Part model, mm, in its own coordinate system. Face numbers are marked on the shaded views. A direction names the side the tool comes from. Coordinates: 2 decimals unless noted, no trailing zeros. Write each loop counter-clockwise with the first axis right and the second up, starting at its lowest first coordinate (ties: lowest second). Pieces come first, ordered by that corner, then holes. Notation, with made-up numbers: (-21, -35.5) - (12, -35.5) arc R17 ccw to (12, -22.5) - close; hole circle Ø3 at (82.5, 65.25). An arc over 180 degrees is marked (long way). Use one line per item in the form item = value. Start each with the question number.
from build123d import *

# Parameters (mm, degrees)
BOSS_EXTRUDE1_OUTLINE_R = 28
BOSS_EXTRUDE1_DEPTH     = 3
BOSS_EXTRUDE3_START     = 20
BOSS_EXTRUDE3_DEPTH     = 20


# Read off the part's stored shape, not the designer's step: Boss-Extrude1
with BuildPart() as part:
    # Boss-Extrude1 outline → Boss-Extrude1 (new body)
    with BuildSketch(Plane.XY):
        with BuildLine():
            Line((30, -70), (30, 0))
            add(Edge.make_bspline(
                [(30, 0), (30, 122.919601085), (65, 122.919601085), (65, 152.5)],
                knots=[0, 0, 0, 0, 1, 1, 1, 1], degree=3))
            ThreePointArc((65, 152.5), (56.213203436, 173.713203436), (35, 182.5))
            add(Edge.make_bspline(
                [(-30, 0), (-30, 182.5), (35, 182.5)],
                knots=[0, 0, 0, 1, 1, 1], degree=2))
            Line((-30, 0), (-30, -70))
            Line((-30, -70), (30, -70))
        make_face()
        with Locations((0, -40)):
            Circle(BOSS_EXTRUDE1_OUTLINE_R, mode=Mode.SUBTRACT)
        with Locations((35, 152.5)):
            Circle(BOSS_EXTRUDE1_OUTLINE_R, mode=Mode.SUBTRACT)
    extrude(amount=BOSS_EXTRUDE1_DEPTH)

    # Sketch3 → Boss-Extrude3 (add)
    with BuildSketch(Plane(origin=(0, 0, 0), x_dir=(-1, 0, 0), z_dir=(0, 0, -1)).offset(BOSS_EXTRUDE3_START)):
        with BuildLine():
            Line((-30, 0), (-30, -70))
            Line((-30, -70), (30, -70))
            Line((30, -70), (30, 0))
            add(Edge.make_bspline(
                [(30, 0), (30, 182.5), (-35, 182.5)],
                knots=[0, 0, 0, 1, 1, 1], degree=2))
            ThreePointArc((-35, 182.5), (-56.213203436, 173.713203436), (-65, 152.5))
            add(Edge.make_bspline(
                [(-65, 152.5), (-65, 122.919601085), (-30, 122.919601085), (-30, 0)],
                knots=[0, 0, 0, 0, 1, 1, 1, 1], degree=3))
        make_face()
        with BuildLine():
            Line((-28, 0), (-28, -68))
            Line((-28, -68), (28, -68))
            Line((28, -68), (28, 0))
            add(Edge.make_bspline(
                [(28, 0), (28, 1.882428306), (27.9894412, 5.668914661), (27.926096555, 13.06867177), (27.76775639, 22.113138456), (27.45115367, 32.600472774), (26.860323994, 46.108658024), (25.805698034, 62.096829622), (24.035349894, 79.847577378), (21.76158749, 96.16063855), (18.061595292, 115.991158762), (12.190733374, 137.171036702), (3.196896645, 156.784444582), (-5.834661566, 168.281935437), (-13.924397363, 174.636152769), (-19.34693601, 177.454327423), (-23.921129202, 179.03154511), (-27.474819646, 179.877405657), (-30.546503211, 180.301515997), (-33.065469046, 180.471580895), (-34.357731157, 180.5), (-35, 180.5)],
                knots=[0.49382409, 0.49382409, 0.49382409, 0.49382409, 0.49393283, 0.494041569, 0.494259049, 0.494476528, 0.494694008, 0.495128967, 0.495563926, 0.495998885, 0.496433844, 0.497303761, 0.498173679, 0.499043597, 0.499478556, 0.499913515, 0.500130995, 0.500348474, 0.500565954, 0.500674693, 0.500783433, 0.500783433, 0.500783433, 0.500783433], degree=3))
            ThreePointArc((-35, 180.5), (-54.798989873, 172.298989873), (-63, 152.5))
            add(Edge.make_bspline(
                [(-63, 152.5), (-63, 152.069757812), (-62.983825045, 151.199286285), (-62.88918488, 149.540019878), (-62.658452593, 147.549741818), (-62.213886299, 145.2784002), (-61.410812146, 142.352354087), (-60.033210568, 138.80365362), (-57.846222702, 134.475175879), (-55.208976195, 129.863823008), (-51.231452034, 123.063969133), (-46.792456906, 114.875371889), (-42.352360132, 104.461715313), (-39.130632465, 95.326409045), (-36.123020534, 84.651250359), (-33.432349584, 72.218369024), (-31.538773259, 60.209244421), (-30.283559802, 49.501788472), (-29.484585221, 40.893227078), (-28.840668199, 31.678686061), (-28.443815603, 23.471810433), (-28.216507678, 16.574966065), (-28.092697498, 11.23438398), (-28.029735078, 6.636857178), (-28.004285655, 2.878237886), (-28, 0.955822894), (-28, 0)],
                knots=[0, 0, 0, 0, 0.015625, 0.03125, 0.0625, 0.09375, 0.125, 0.1875, 0.25, 0.3125, 0.375, 0.5, 0.5625, 0.625, 0.6875, 0.75, 0.8125, 0.84375, 0.875, 0.90625, 0.9375, 0.953125, 0.96875, 0.984375, 0.9921875, 1, 1, 1, 1], degree=3))
        make_face(mode=Mode.SUBTRACT)
    extrude(amount=-BOSS_EXTRUDE3_DEPTH)


solid = part.part
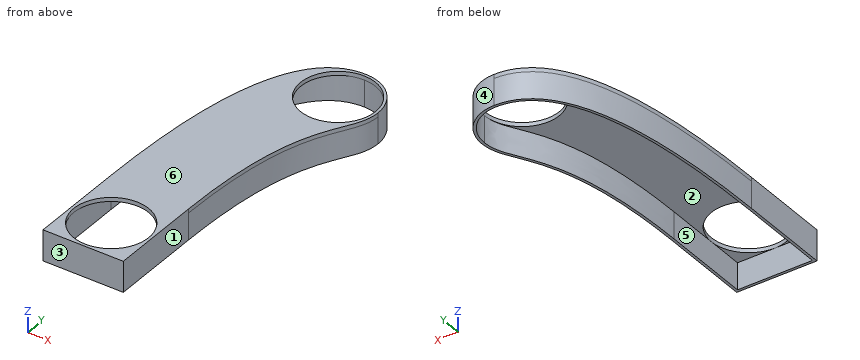
Q1. Which spindle directions (+Z, -Z, +X, -X, +Y, -Y) get a long thin tool onto all of the face, cutting with end or side? Do the marked faces 1, 2 and 3. Say none if no direction does.
Q2. Slice it at B-B (x = 22.5). Count the separate pieces of the cut face and the enclosed holes in it, plus the area to 3 significant figures.
Q3. Mould opens along X. For the marked faces 4, 5 and 6 say: released by +X, released by -X, zero draft, split by the parting line, or undercut.
Q4. Slice it at A-A (y = -14.5). List the corners of the cut face in (x, z), plus the area to 3 significant figures.
Q5. Pin check, flat tips, straight feed: P1, Ø6, axis at y = -33, z = -7.5, coming from the +X side; P2, Ø5, axis at x = 40.5, z = -5.5, coming from the +Y side; P3, Ø3, axis at x = 7.5, z = -15, coming from the +Y side. Stop position of each tip, or through.
Q6. Drill centre lines: probe 1 along X at (y, z) = (-4.5, -7.75); probe 2 along Z at (x, y) = (0.5, 79); probe 3 along Y at (x, z) = (55.5, -16.5). Where is each one in solid material? Low to high.
Solution:
q1.face_1 = +Z, -Z, +X, -Y
q1.face_2 = -Z
q1.face_3 = +Z, -Z, +X, -X, -Y
q2.separate_pieces = 3
q2.enclosed_holes = 0
q2.area = 584 mm2
q3.face_4 = released by +X
q3.face_5 = undercut
q3.face_6 = zero draft
q4.outline = (-30, -20) - (-28, -20) - (-28, 0) - (-11.57, 0) - (-11.57, 3) - (-30, 3) - close; (11.57, 0) - (28, 0) - (28, -20) - (30, -20) - (30, 3) - (11.57, 3) - close
q4.area = 191 mm2
q5.P1 = 30
q5.P2 = 182.35
q5.P3 = 173.23
q6.probe_1 = -30 to -28, 28 to 30
q6.probe_2 = 0 to 3
q6.probe_3 = 126.4 to 130.39, 171.57 to 174.4
